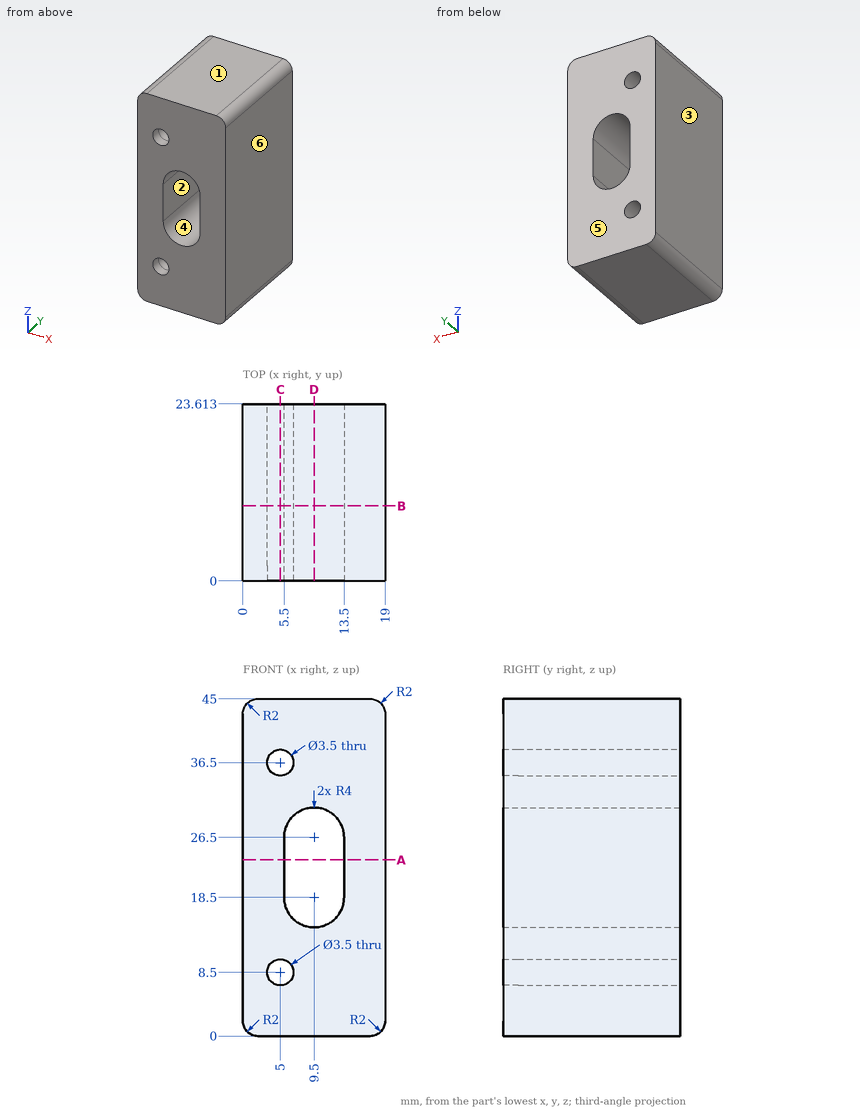
Geometry check sheet. Reference: drawing and pictorial views, mm from the part's lowest x, y, z. A direction names the side the tool comes from. Round coordinates to 2 decimals unless told otherwise and drop trailing zeros. Write each loop counter-clockwise with the first axis right and the second up, starting at its lowest first coordinate (ties: lowest second). Pieces come first, ordered by that corner, then holes.
(1) Section check C-C (x = 5). Enter the section's corners in (y, z), plus the area to 3 significant figures.
Returned:
outline: (0, 0) - (23.61, 0) - (23.61, 6.75) - (0, 6.75) - close; (0, 10.25) - (23.61, 10.25) - (23.61, 34.75) - (0, 34.75) - close; (0, 38.25) - (23.61, 38.25) - (23.61, 45) - (0, 45) - close
area: 897 mm2
(2) Depth check by flat-ended pin: pin 1 Ø2 at (x, z) = (5, 36.5) entering from -Y. Enter the tip coordinate at first touch or a pass-through.
Returned:
pin 1: passes through
(3) Material ranges on line 1 (Z direction, x = 5, y = 0.8); line 2 (X direction, y = 0.4, z = 36.5); line 3 (X direction, y = 9, z = 23.5), recorded low to high.
Returned:
line 1: z = 0 to 6.75, 10.25 to 34.75, 38.25 to 45
line 2: x = 0 to 3.25, 6.75 to 19
line 3: x = 0 to 5.5, 13.5 to 19
(4) Section check A-A (z = 23.5). Enter the section's corners in (x, y).
Returned:
outline: (0, 0) - (5.5, 0) - (5.5, 23.61) - (0, 23.61) - close; (13.5, 0) - (19, 0) - (19, 23.61) - (13.5, 23.61) - close
(5) Access from +Z, -Z, +X, -X, +Y, -Y to the whole of each face (thin tool, end or side, straight path). Record for the marked faces 1 and 2.
Returned:
face 1: +Z, +X, -X, +Y, -Y
face 2: +Y, -Y
(6) Section check D-D (x = 9.5). Enter the section's corners in (y, z).
Returned:
outline: (0, 0) - (23.61, 0) - (23.61, 14.5) - (0, 14.5) - close; (0, 30.5) - (23.61, 30.5) - (23.61, 45) - (0, 45) - close
(7) Section check B-B (y = 10). Enter the section's corners in (x, z), plus the area to 3 significant figures.
Returned:
outline: (0, 2) arc R2 ccw to (2, 0) - (17, 0) arc R2 ccw to (19, 2) - (19, 43) arc R2 ccw to (17, 45) - (2, 45) arc R2 ccw to (0, 43) - close; hole circle Ø3.5 at (5, 8.5); hole circle Ø3.5 at (5, 36.5); hole (5.5, 18.5) arc R4 ccw to (13.5, 18.5) - (13.5, 26.5) arc R4 ccw to (5.5, 26.5) - close
area: 718 mm2
(8) Mould release check, pull along X, two halves, no side actions. Record for the marked faces 3, 4, 5 and 6: pulls with the +X half, pulls with the -X half, needs draft (parallel to the pull), parting line crosses it, or undercut.
Returned:
face 3: pulls with the -X half
face 4: undercut
face 5: needs draft
face 6: pulls with the +X half
